Work out the finished part from the listing and answer in its coordinate system (mm). Face numbers are marked on the shaded views. A direction names the side the tool comes from. Coordinates: 2 decimals unless noted, no trailing zeros. Write each loop counter-clockwise with the first axis right and the second up, starting at its lowest first coordinate (ties: lowest second). Pieces come first, ordered by that corner, then holes. Notation, with made-up numbers: M 43,-31 L 60,-31 A26 ccw 60,-11 Z; hole C 26.25,14.25 d5. An arc over 180 degrees is marked long. Answer as CSV lines item,"result". Start each with the question number.
(1) A cutting plane is placed at D-D on y = 3.25. Give the vertices of the cut face in (x, z), then the cut area to 3 significant figures.
(2) A cutting plane is placed at C-C on z = 21.25. Give the vertices of the cut face in (x, y), then the cut area to 3 significant figures.
(3) A cutting plane is placed at A-A on x = 0. Give the vertices of the cut face in (y, z).
(4) For the marked faces 1 and 2, determine the directions among +Z, -Z, +X, -X, +Y, -Y from which every point of the face is accessible in a straight line to the end or side of a thin tool.
(5) Flat-ended cylindrical pins translate along their axes: P1, Ø4, axis at x = -2.5, z = 7, coming from the -Y side; P2, Ø1.5, axis at y = 2, z = 18, coming from the -X side; P3, Ø6, axis at y = 4, z = 17, coming from the +X side. Find the tip coordinate at first contact, or state that the pin passes through.
(6) Find the intervals of material crossed by L1, parallel to Y at x = 0, z = 18; L2, parallel to Y at x = 0, z = 4.5; L3, parallel to Z at x = 0, y = 3.5, in increasing order. Write a range as [from, to].
(7) The mould has two halves that part along X. Classify the marked faces 3, 4 and 5: released by +X, released by -X, zero draft, split by the parting line, or undercut.
(8) A cutting plane is placed at B-B on y = 0. Give the vertices of the cut face in (x, z), then the cut area to 3 significant figures.
from build123d import *

# Parameters (mm, degrees)
SKETCH_1_R          = 5
EXTRUDE_1_DEPTH     = 23
CUT_EXTRUDE_1_DEPTH = 10
SKETCH_3_R          = 4
CUT_EXTRUDE_2_DEPTH = 13


with BuildPart() as part:
    # 草图1 → 凸台-拉伸1 (new body)
    with BuildSketch(Plane.XY):
        Circle(SKETCH_1_R)
    extrude(amount=EXTRUDE_1_DEPTH)

    # 草图2 → 切除-拉伸1 (cut)
    with BuildSketch(Plane.XY.offset(23)):
        with BuildLine():
            Line((-2.236067977, 2), (2.236067977, 2))
            ThreePointArc((2.236067977, 2), (0, -3), (-2.236067977, 2))
        make_face()
    extrude(amount=-CUT_EXTRUDE_1_DEPTH, mode=Mode.SUBTRACT)

    # 草图3 → 切除-拉伸2 (cut)
    with BuildSketch(Plane(origin=(0, 0, 0), x_dir=(-1, 0, 0), z_dir=(0, 0, -1))):
        Circle(SKETCH_3_R)
    extrude(amount=-CUT_EXTRUDE_2_DEPTH, mode=Mode.SUBTRACT)


solid = part.part
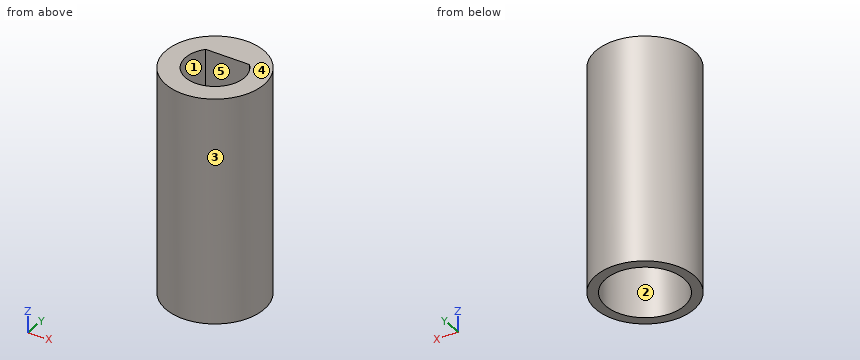
Here are the results:
1,outline,"M -3.8,0 L -2.33,0 L -2.33,13 L 2.33,13 L 2.33,0 L 3.8,0 L 3.8,23 L -3.8,23 Z"
1,area,"114 mm^2"
2,outline,"C 0,0 d10; hole M -2.24,2 A3 ccw long 2.24,2 Z"
2,area,"53.4 mm^2"
3,outline,"M -5,0 L -4,0 L -4,13 L -3,13 L -3,23 L -5,23 Z; M 2,13 L 4,13 L 4,0 L 5,0 L 5,23 L 2,23 Z"
4,face 1,"+Z, -Z"
4,face 2,"-Z"
5,P1,"stops at y = -4.97"
5,P2,"stops at x = -4.84"
5,P3,"stops at x = 4.9"
6,L1,"y = [-5, -3], [2, 5]"
6,L2,"y = [-5, -4], [4, 5]"
6,L3,"z = [13, 23]"
7,face 3,"split by the parting line"
7,face 4,"zero draft"
7,face 5,"undercut"
8,outline,"M -5,0 L -4,0 L -4,13 L -3,13 L -3,23 L -5,23 Z; M 3,13 L 4,13 L 4,0 L 5,0 L 5,23 L 3,23 Z"
8,area,"66.0 mm^2"
